```python
from build123d import *

# Parameters (mm, degrees)
SKETCH_1_R             = 5.4
EXTRUDE_1_DEPTH        = 67
CHAMFER_1_SIZE         = 0.5
SKETCH_2_R             = 3.3
EXTRUDE_2_DEPTH        = 8
HOLE_WIZARD_M5_1_D     = 4.2
HOLE_WIZARD_M5_1_DEPTH = 12.4
HOLE_WIZARD_M5_1_TIP   = 1.2618073
CHAMFER_3_SIZE         = 0.5
SKETCH_5_W             = 10
SKETCH_5_H             = 3
CUT_EXTRUDE_3_DEPTH    = 13
CHAMFER_4_SIZE         = 0.5


with BuildPart() as part:
    # 草图1 → 拉伸1 (new body)
    with BuildSketch(Plane.XY):
        Circle(SKETCH_1_R)
    extrude(amount=EXTRUDE_1_DEPTH)

    # 倒角1
    chamfer_1_edges = [part.edges().sort_by_distance(p)[0] for p in [
        (-5.4, 0, 0),
        (-5.4, 0, 67),
    ]]
    chamfer(chamfer_1_edges, length=CHAMFER_1_SIZE)

    # 草图2 → 拉伸2 (add)
    with BuildSketch(Plane.XY.offset(67)):
        Circle(SKETCH_2_R)
    extrude(amount=EXTRUDE_2_DEPTH)

    # M5 螺纹孔1
    with Locations(Plane(origin=(0, 0, 0), x_dir=(-1, 0, 0), z_dir=(0, 0, -1))):
        with Locations((0, 0)):
            Hole(HOLE_WIZARD_M5_1_D / 2, depth=HOLE_WIZARD_M5_1_DEPTH)
            with Locations((0, 0, -(HOLE_WIZARD_M5_1_DEPTH + HOLE_WIZARD_M5_1_TIP / 2))):  # 118° drill point
                Cone(0, HOLE_WIZARD_M5_1_D / 2, HOLE_WIZARD_M5_1_TIP, mode=Mode.SUBTRACT)

    # 倒角3
    chamfer_3_edges = [part.edges().sort_by_distance(p)[0] for p in [
        (-2.1, 0, 0),
    ]]
    chamfer(chamfer_3_edges, length=CHAMFER_3_SIZE)

    # 草图5 → 拉伸3 (cut)
    with BuildSketch(Plane.XY):
        with Locations((0, 6.5)):
            Rectangle(SKETCH_5_W, SKETCH_5_H)
    cut_extrude_3 = extrude(amount=CUT_EXTRUDE_3_DEPTH, mode=Mode.SUBTRACT)

    # 镜向1: 拉伸3 across plane
    add(cut_extrude_3.mirror(Plane.ZX), mode=Mode.SUBTRACT)

    # 倒角4
    chamfer_4_edges = [part.edges().sort_by_distance(p)[0] for p in [
        (-3.3, 0, 67),
    ]]
    chamfer(chamfer_4_edges, length=CHAMFER_4_SIZE)


solid = part.part
```
Could you check a few things on this model? Use its own coordinates, in mm. A direction names the side the tool comes from. Give positions to 0.01 mm unless a question says otherwise; leave off trailing zeros. Order: outer loops, then holes, each group sorted by start corner. A loop starts at its lowest first (then second) coordinate and runs counter-clockwise, first axis right, second up.
Q1. For faces 4 (the cylindrical face through (-2.43, 2.23, 71.2)), 5 (the cylindrical face through (2.003, 0.631, 6.533)), 6 (the flat face through (0, 5, 6)), which set-ups out of +Z, -Z, +X, -X, +Y, -Y let a thin tool reach every point of the face, with its end or its side?
Q2. If I drill on line 1 along X through (y, z) = (0, 7.25); line 2 along Y through (x, z) = (0, 5); line 3 along Y through (x, z) = (-0.25, 69.5), over which ranges is the centre line in solid material (lowest first)?
Q3. Suppose I cut it at A-A, the plane z = 17.5. Write out the boundary of the cut face in (x, y).
Q4. I'm going to push flat-ended pins straight in: P1, Ø2, axis at x = -1, z = 4.5, coming from the -Y side; P2, Ø1, axis at y = 4, z = 50.5, coming from the -X side; P3, Ø2, axis at x = -4, z = 44, coming from the +Y side. Where does each tip first touch, or does it pass through?
Q5. We'd pull the mould along X, two halves only. Please class faces 1 (the flat face through (0, -5, 6)), 2 (the conical face through (-0.35, 0.11, 13.44)), 3 (the cylindrical face through (5.15, 1.62, 33.04)): +X half, -X half, draft (parallel to the pull), parting line (faces both ways), or undercut.
Solution:
1. face 4: +Z
1. face 5: -Z
1. face 6: -Z, +X, -X, +Y
2. line 1: x = -5.4 to -2.1, 2.1 to 5.4
2. line 2: y = -5 to -2.1, 2.1 to 5
2. line 3: y = -3.29 to 3.29
3. outline: circle Ø10.8 at (0, 0)
4. P1: stops at y = -5
4. P2: stops at x = -4.11
4. P3: stops at y = 4.49
5. face 1: draft
5. face 2: undercut
5. face 3: parting line
